Autodesk Inventor part; units mm, degrees
ref_plane "YZ Plane" through (0, 0, 0) normal (1, 0, 0) x (0, 1, 0)
ref_plane "XZ Plane" through (0, 0, 0) normal (0, 1, 0) x (-1, 0, 0)
ref_plane "XY Plane" through (0, 0, 0) normal (0, 0, 1) x (1, 0, 0)
sketch "Sketch1" plane through (0, 0, 0) normal (1, 0, 0) x (0, 1, 0)
  line L0 (10.5, -1) -> (9.5, -1)
  line L1 (9.5, -1) -> (9.5, -40)
  line L2 (9.5, -40) -> (10.5, -40)
  line L3 (10.5, -40) -> (10.5, -1)
  line L4 (14.5, -40) -> (8.5, -40)
  line L5 (8.5, -40) -> (8.5, -41)
  line L6 (8.5, -41) -> (14.5, -41)
  line L7 (14.5, -41) -> (14.5, -40)
  line L8 (0, -49.2) -> (0, 8.2)
  point P0 (0, 0)
  dimension "d0" = 1
  dimension "d1" = 1
  dimension "d2" = 1
  dimension "d3" = 10.5
  dimension "d4" = 4
  dimension "d5" = 40
revolve "Revolution1" add sketch "Sketch1" angle 360 about axis through (0, 0, -10) along (0, 0, 1)
thread "Thread1"
properties part number "bearingShellInner"
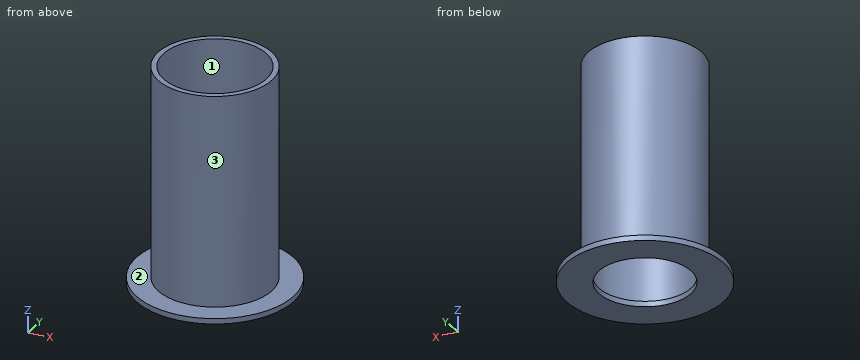
For this review, take the finished solid that the model builds, in its own axes (mm). Face numbers are marked on the shaded views. Coordinates: 2 decimals unless noted, no trailing zeros. Order: outer loops, then holes, each group sorted by start corner. A loop starts at its lowest first (then second) coordinate and runs counter-clockwise, first axis right, second up. Notation, with made-up numbers: (77, -22.5) -> (112, -22.5) arc R25 ccw to (112, -3.5) -> close; hole circle Ø10 at (-32, -9). An arc over 180 degrees is marked (long way). Return JSON: item names as keys, results as strings.
1. We need section D-D on y = -12.5. Write out the cut boundary in (x, z), and give its area (3 significant figures).
Answer block:
{"outline": "(-7.35, -41) -> (7.35, -41) -> (7.35, -40) -> (-7.35, -40) -> close", "area": "14.7 mm²"}
2. We need section A-A on y = 0. Write out the cut boundary in (x, z).
Answer block:
{"outline": "(-14.5, -41) -> (-8.5, -41) -> (-8.5, -40) -> (-9.5, -40) -> (-9.5, -1) -> (-10.5, -1) -> (-10.5, -40) -> (-14.5, -40) -> close; (8.5, -41) -> (14.5, -41) -> (14.5, -40) -> (10.5, -40) -> (10.5, -1) -> (9.5, -1) -> (9.5, -40) -> (8.5, -40) -> close"}
3. For line 1 (X direction, y = 0, z = -40.25); line 2 (X direction, y = 0.25, z = -36), list the stretches that pass through material, from the lowest coordinate up. Write a range as from..to.
Answer block:
{"line 1": "-14.5..-8.5, 8.5..14.5", "line 2": "-10.5..-9.5, 9.5..10.5"}
4. For pin 1 Ø1 at (y, z) = (3.5, -10) entering from -X; pin 2 Ø1 at (y, z) = (-5, -28.5) entering from +X; pin 3 Ø8 at (x, y) = (-8.5, 4) entering from +Z; pin 4 Ø1 at (x, y) = (10.5, 8) entering from +Z, all flat-tipped, find the tip position at first contact; note any pin that passes through.
Answer block:
{"pin 1": "x = -10.06", "pin 2": "x = 9.49", "pin 3": "z = -1", "pin 4": "z = -40"}
5. The part is to be moulded in two halves that separate along Y. For the marked faces 1, 2 and 3, say which applies: +Y half, -Y half, draft (parallel to the pull), parting line (faces both ways), or undercut.
Answer block:
{"face 1": "undercut", "face 2": "draft", "face 3": "parting line"}
6. We need section C-C on z = -13.5. Write out the cut boundary in (x, y), and give its area (3 significant figures).
Answer block:
{"outline": "circle Ø21 at (0, 0); hole circle Ø19 at (0, 0)", "area": "62.8 mm²"}
